Here's how the part is built. I have some questions about the finished solid (model axes, mm). A direction names the side the tool comes from. Round coordinates to 2 decimals unless told otherwise and drop trailing zeros. Write each loop counter-clockwise with the first axis right and the second up, starting at its lowest first coordinate (ties: lowest second). Pieces come first, ordered by that corner, then holes. Notation, with made-up numbers: (-4, 85.25) - (11, 85.25) arc R13 ccw to (11, 108.25) - close; hole circle Ø9 at (-11.5, -32). An arc over 180 degrees is marked (long way). One line per item, written item: value. Start each with the question number.
Item 1: Imagine slicing it at A-A, the plane z = -2937.5. Please give me the cut outline in (x, y).
Item 2: For faces 1 (the face through (-699, 107, -3100)), 2 (the face through (-691.96, 53, -2957)), 3 (the face through (-696.087, 65, -3042)), which set-ups out of +Z, -Z, +X, -X, +Y, -Y let a thin tool reach every point of the face, with its end or its side?
Item 3: Imagine slicing it at B-B, the plane y = 44. Please give me the cut outline in (x, z) (1 decimal).
Item 4: Imagine slicing it at D-D, the plane y = 9. Please give me the cut outline in (x, z) (1 decimal).
Item 5: Imagine slicing it at C-C, the plane x = -715.5. Please give me the cut outline in (y, z) (3 decimals).
Item 6: For P1, Ø4.5, axis at x = -794.5, z = -3020.5, coming from the +Y side; P2, Ø3, axis at x = -709.5, z = -3016, coming from the +Y side; P3, Ø4, axis at x = -699, y = 66, coming from the +Z side, each with a flat end and sliding along its axis, tell me the tip position at first contact or that it passes through.
Item 7: Thinking about a two-plate mould opening in Z: for faces 4 (the face through (-749, 53, -3167.3)), 5 (the face through (-749, -3, -3043)), 6 (the face through (-795.5, 22.31, -3041.07)), 7 (the face through (-695.7, 40.9, -2990.596)), which applies, released by +Z, released by -Z, zero draft, split by the parting line, or undercut?
Item 8: If I drill on line 1 (X direction, y = 50, z = -3142); line 2 (X direction, y = 79.5, z = -3034.5); line 3 (Y direction, x = -715, z = -3130), over which ranges is the centre line in solid material (lowest first)?
```python
from build123d import *

# Parameters (mm, degrees)
BOSS_EXTRUDE1_DEPTH = 107
SKETCH7_W           = 122.268
SKETCH7_H           = 249.395
BOSS_EXTRUDE2_DEPTH = 3
SKETCH8_W           = 9.0805
SKETCH8_H           = 57.785
BOSS_EXTRUDE3_DEPTH = 30
CUT_EXTRUDE1_DEPTH  = 9.0805
CUT_EXTRUDE2_DEPTH  = 9.0805
FILLET1_R           = 2
CUT_EXTRUDE3_DEPTH  = 3271.793089872


with BuildPart() as part:
    # Sketch6 → Boss-Extrude1 (new body)
    with BuildSketch(Plane(origin=(0, 0, 0), x_dir=(1, 0, 0), z_dir=(0, 1, 0))):
        Polygon((-809.2275, 2922.905), (-804.2275, 2922.905), (-804.2275, 2990.596), (-800.1, 2990.596), (-800.1, 3162.3), (-701.04, 3162.3), (-701.04, 3092.958), (-696.087, 3092.958), (-696.087, 2990.596), (-691.9595, 2990.596), (-691.9595, 2922.905), (-686.9595, 2922.905), (-686.9595, 3167.3), (-809.2275, 3167.3), align=None)
    extrude(amount=BOSS_EXTRUDE1_DEPTH)

    # Sketch7 → Boss-Extrude2 (add)
    with BuildSketch(Plane.XZ):
        with Locations((-748.0935, -3042.6025)):
            Rectangle(SKETCH7_W, SKETCH7_H)
    extrude(amount=BOSS_EXTRUDE2_DEPTH)

    # Sketch8 → Boss-Extrude3 (add)
    with BuildSketch(Plane(origin=(0, 0, 0), x_dir=(1, 0, 0), z_dir=(0, 1, 0))):
        with Locations((-795.55975, 3019.4885)):
            Rectangle(SKETCH8_W, SKETCH8_H)
        with Locations((-700.62725, 3019.4885)):
            Rectangle(SKETCH8_W, SKETCH8_H)
    extrude(amount=BOSS_EXTRUDE3_DEPTH)

    # Sketch9 → Cut-Extrude1 (cut)
    with BuildSketch(Plane(origin=(-791.0195, 0, 0), x_dir=(0, 0, -1), z_dir=(1, 0, 0))):
        Polygon((2990.596, 30), (2990.596, 15), (3005.596, 30), align=None)
        Polygon((3048.381, 30), (3033.381, 30), (3048.381, 15), align=None)
    extrude(amount=-CUT_EXTRUDE1_DEPTH, mode=Mode.SUBTRACT)

    # Sketch10 → Cut-Extrude2 (cut)
    with BuildSketch(Plane.ZY.offset(705.1675)):
        Polygon((-3048.381, 30), (-3048.381, 15), (-3033.381, 30), align=None)
        Polygon((-2990.596, 30), (-3005.596, 30), (-2990.596, 15), align=None)
    extrude(amount=-CUT_EXTRUDE2_DEPTH, mode=Mode.SUBTRACT)

    # Fillet1
    fillet1_edges = [part.edges().sort_by_distance(p)[0] for p in [
        (-795.55975, 30, -3005.596),
        (-795.55975, 30, -3033.381),
        (-700.62725, 30, -3033.381),
        (-700.62725, 30, -3005.596),
        (-809.2275, 53.5, -2922.905),
        (-809.2275, 52, -3167.3),
        (-686.9595, 52, -3167.3),
        (-686.9595, 53.5, -2922.905),
    ]]
    fillet(fillet1_edges, radius=FILLET1_R)

    # Sketch11 → Cut-Extrude3 (cut, through all)
    with BuildSketch(Plane(origin=(0, 0, 0), x_dir=(-1, 0, 0), z_dir=(0, 1, 0))):
        with BuildLine():
            Line((804.2275, -2922.905), (691.9595, -2922.905))
            Line((691.9595, -2922.905), (688.9595, -2922.905))
            ThreePointArc((688.9595, -2922.905), (687.545286438, -2923.490786438), (686.9595, -2924.905))
            Line((686.9595, -2924.905), (686.9595, -2917.905))
            Line((686.9595, -2917.905), (809.2275, -2917.905))
            Line((809.2275, -2917.905), (809.2275, -2924.905))
            ThreePointArc((809.2275, -2924.905), (808.641713562, -2923.490786438), (807.2275, -2922.905))
            Line((807.2275, -2922.905), (804.2275, -2922.905))
        make_face()
    extrude(amount=-CUT_EXTRUDE3_DEPTH, mode=Mode.SUBTRACT)


solid = part.part
```
Values follow:
1. outline: (-809.23, -3) - (-686.96, -3) - (-686.96, 107) - (-691.96, 107) - (-691.96, 0) - (-804.23, 0) - (-804.23, 107) - (-809.23, 107) - close
2. face 1: +Z, -Z, +X, -X, +Y
2. face 2: +Z, +Y
2. face 3: +Y
3. outline: (-809.2, -3165.3) arc R2 ccw to (-807.2, -3167.3) - (-689, -3167.3) arc R2 ccw to (-687, -3165.3) - (-687, -2924.9) arc R2 ccw to (-689, -2922.9) - (-692, -2922.9) - (-692, -2990.6) - (-696.1, -2990.6) - (-696.1, -3093) - (-701, -3093) - (-701, -3162.3) - (-800.1, -3162.3) - (-800.1, -2990.6) - (-804.2, -2990.6) - (-804.2, -2922.9) - (-807.2, -2922.9) arc R2 ccw to (-809.2, -2924.9) - close
4. outline: (-809.2, -3165.3) arc R2 ccw to (-807.2, -3167.3) - (-689, -3167.3) arc R2 ccw to (-687, -3165.3) - (-687, -2924.9) arc R2 ccw to (-689, -2922.9) - (-692, -2922.9) - (-692, -2990.6) - (-705.2, -2990.6) - (-705.2, -3048.4) - (-696.1, -3048.4) - (-696.1, -3093) - (-701, -3093) - (-701, -3162.3) - (-800.1, -3162.3) - (-800.1, -3048.4) - (-791, -3048.4) - (-791, -2990.6) - (-804.2, -2990.6) - (-804.2, -2922.9) - (-807.2, -2922.9) arc R2 ccw to (-809.2, -2924.9) - close
5. outline: (-3, -3167.3) - (107, -3167.3) - (107, -3162.3) - (0, -3162.3) - (0, -2922.905) - (-3, -2922.905) - close
6. P1: stops at y = 30
6. P2: stops at y = 0
6. P3: stops at z = -3092.96
7. face 4: released by -Z
7. face 5: zero draft
7. face 6: undercut
7. face 7: released by +Z
8. line 1: x = -809.23 to -800.1, -701.04 to -686.96
8. line 2: x = -809.23 to -800.1, -696.09 to -686.96
8. line 3: y = -3 to 0
